For this review, take the finished solid that the model builds, in its own axes (mm). Round coordinates to 2 decimals unless told otherwise and drop trailing zeros. Loops run counter-clockwise (first coordinate to the right, second up) from the corner with the lowest first, then second, coordinate; pieces in that order, holes last. Notation, with made-up numbers: (-36.75, 69.25) -> (-6.75, 69.25) arc R27 ccw to (-6.75, 98.25) -> close; hole circle Ø5 at (-35, -14). An arc over 180 degrees is marked (long way). Write each question's results on one line, items separated by ' | '.
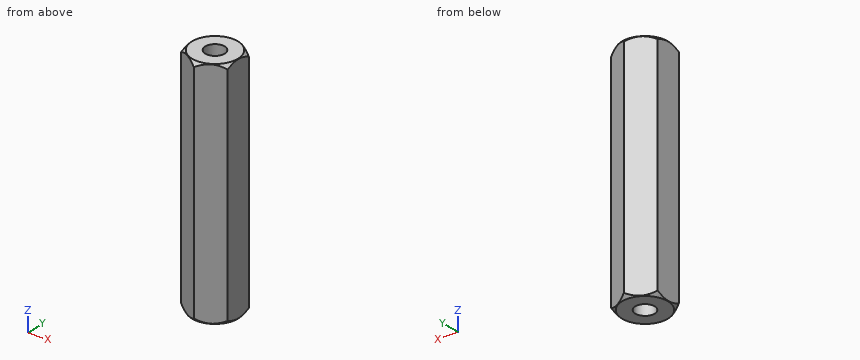
```python
from build123d import *

# Parameters (mm, degrees)
SALIENTE_EXTRUIR1_DEPTH = 15
CROQUIS3_R              = 1.25
CORTAR_EXTRUIR1_DEPTH   = 30


with BuildPart() as part:
    # Croquis1 → Saliente-Extruir1 (new body, symmetric)
    with BuildSketch(Plane.XY):
        Polygon((0, 3.464101615), (-3, 1.732050808), (-3, -1.732050808), (0, -3.464101615), (3, -1.732050808), (3, 1.732050808), align=None)
    extrude(amount=SALIENTE_EXTRUIR1_DEPTH, both=True)

    # Croquis2 → Cortar-Revolución2 (revolve, cut)
    with BuildSketch(Plane(origin=(0, 0, 0), x_dir=(0, 0, -1), z_dir=(1, 0, 0))):
        Polygon((15, 2.964101615), (19.5, 2.964101615), (19.5, 7.964101615), (14.5, 7.964101615), (14.5, 3.464101615), align=None)
        Polygon((-19.5, 2.964101615), (-19.5, 7.964101615), (-14.5, 7.964101615), (-14.5, 3.464101615), (-15, 2.964101615), align=None)
    revolve(axis=Axis((0, 0, 17.803147854), (0, 0, -1)), mode=Mode.SUBTRACT)

    # Croquis3 → Cortar-Extruir1 (cut)
    with BuildSketch(Plane.XY.offset(15)):
        Circle(CROQUIS3_R)
    extrude(amount=-CORTAR_EXTRUIR1_DEPTH, mode=Mode.SUBTRACT)


solid = part.part
```
1. To check wall thickness, follow probe 1 along X at (y, z) = (1, 12); probe 2 along X at (y, z) = (-0.75, 10); probe 3 along Y at (x, z) = (0.95, -3). State the ranges of each line that lie inside material, in increasing order.
Values found:
probe 1: x = -3 to -0.75, 0.75 to 3 | probe 2: x = -3 to -1, 1 to 3 | probe 3: y = -2.92 to -0.81, 0.81 to 2.92
2. Consider section B-B (y = 0). State the section outline as (x, z) points, plus the area to 3 significant figures.
Values found:
outline: (-3, -14.96) -> (-2.96, -15) -> (-1.25, -15) -> (-1.25, 15) -> (-2.96, 15) -> (-3, 14.96) -> close; (1.25, -15) -> (2.96, -15) -> (3, -14.96) -> (3, 14.96) -> (2.96, 15) -> (1.25, 15) -> close | area: 105 mm2
3. Consider section A-A (z = -5). State the section outline as (x, y) points, plus the area to 3 significant figures.
Values found:
outline: (-3, -1.73) -> (0, -3.46) -> (3, -1.73) -> (3, 1.73) -> (0, 3.46) -> (-3, 1.73) -> close; hole circle Ø2.5 at (0, 0) | area: 26.3 mm2
